Verification items for the finished model (mm, model axes). A direction names the side the tool comes from. Give positions to 0.01 mm unless a question says otherwise; leave off trailing zeros. Loops run counter-clockwise (first coordinate to the right, second up) from the corner with the lowest first, then second, coordinate; pieces in that order, holes last. Notation, with made-up numbers: M 64.5,81 L 99.5,81 A6 ccw 99.5,89 Z; hole C 15.5,6.25 d3. An arc over 180 degrees is marked long. Use a Markdown table: item, result.
from build123d import *

# Parameters (mm, degrees)
SKETCH1_W           = 30
SKETCH1_H           = 30
BOSS_EXTRUDE1_DEPTH = 150
SKETCH2_R           = 12.5
CUT_EXTRUDE1_DEPTH  = 120
SKETCH3_W           = 10
SKETCH3_H           = 5
BOSS_EXTRUDE2_DEPTH = 15
SKETCH4_R           = 2.5
CUT_EXTRUDE2_DEPTH  = 10


with BuildPart() as part:
    # Sketch1 → Boss-Extrude1 (new body)
    with BuildSketch(Plane.XY):
        with Locations((-15, 15)):
            Rectangle(SKETCH1_W, SKETCH1_H)
    extrude(amount=BOSS_EXTRUDE1_DEPTH)

    # Sketch2 → Cut-Extrude1 (cut)
    with BuildSketch(Plane.XY.offset(150)):
        with Locations((-14.468504341, 15)):
            Circle(SKETCH2_R)
    extrude(amount=-CUT_EXTRUDE1_DEPTH, mode=Mode.SUBTRACT)

    # Sketch3 → Boss-Extrude2 (add)
    with BuildSketch(Plane(origin=(0, 0, 0), x_dir=(-1, 0, 0), z_dir=(0, 0, -1))):
        with Locations((15, 15)):
            Rectangle(SKETCH3_W, SKETCH3_H)
    extrude(amount=BOSS_EXTRUDE2_DEPTH)

    # Sketch4 → Cut-Extrude2 (cut)
    with BuildSketch(Plane.XZ.offset(-12.5)):
        with Locations(Location((-15, -10, 0), (0, 0, 270))):
            Circle(SKETCH4_R)
    extrude(amount=-CUT_EXTRUDE2_DEPTH, mode=Mode.SUBTRACT)


solid = part.part
(1) Material ranges on line 1 (X direction, y = 15.4, z = -10); line 2 (X direction, y = 16.5, z = 124.5); line 3 (Y direction, x = -16.75, z = -7.5), recorded low to high.
Results below:
| item | result |
|---|---|
| line 1 | -20 to -17.5, -12.5 to -10 |
| line 2 | -30 to -26.88, -2.06 to 0 |
| line 3 | 12.5 to 17.5 |
(2) Cross-section at C-C on x = -15. Record the cut outline in (y, z), then the cut area to 3 significant figures.
Results below:
| item | result |
|---|---|
| outline | M 0,0 L 12.5,0 L 12.5,-7.5 L 17.5,-7.5 L 17.5,0 L 30,0 L 30,150 L 27.49,150 L 27.49,30 L 2.51,30 L 2.51,150 L 0,150 Z; M 12.5,-15 L 17.5,-15 L 17.5,-12.5 L 12.5,-12.5 Z |
| area | 1,550 mm^2 |
(3) Draft check along Y on faces 5 (the flat face through (-15, 17.5, -7)), 6 (the cylindrical face through (-2.922, 10.212, 90.84)), 7 (the flat face through (-15, 15, -15)). Enter one of: +Y half, -Y half, draft (parallel to the pull), parting line (faces both ways), or undercut.
Results below:
| item | result |
|---|---|
| face 5 | +Y half |
| face 6 | undercut |
| face 7 | draft |
(4) Set-up check for faces 1 (the flat face through (-15, 12.5, -7)), 2 (the flat face through (-15, 15, 30)), 3 (the flat face through (-20, 15, -7)), 4 (the flat face through (-10, 15, -7)): record each of +Z, -Z, +X, -X, +Y, -Y from which the full face is reachable in a straight line by a thin tool's end or side.
Results below:
| item | result |
|---|---|
| face 1 | -Z, +X, -X, -Y |
| face 2 | +Z |
| face 3 | -Z, -X, +Y, -Y |
| face 4 | -Z, +X, +Y, -Y |
(5) Gauge pin test, flat ends, axial feed: P1, Ø2.5, axis at y = 15.5, z = -8.5, coming from the -X side; P2, Ø5, axis at x = -13.5, z = -11, coming from the +Y side; P3, Ø3, axis at x = -4, y = 12.5, coming from the -Z side. Record the tip position at first contact, or that the pin passes through.
Results below:
| item | result |
|---|---|
| P1 | x = -20 |
| P2 | y = 17.5 |
| P3 | z = 0 |
(6) Cross-section at D-D on z = 59.5. Record the cut outline in (x, y), then the cut area to 3 significant figures.
Results below:
| item | result |
|---|---|
| outline | M -30,0 L 0,0 L 0,30 L -30,30 Z; hole C -14.47,15 d25 |
| area | 409 mm^2 |
(7) Cross-section at B-B on z = -10. Record the cut outline in (x, y).
Results below:
| item | result |
|---|---|
| outline | M -20,12.5 L -17.5,12.5 L -17.5,17.5 L -20,17.5 Z; M -12.5,12.5 L -10,12.5 L -10,17.5 L -12.5,17.5 Z |
(8) Cross-section at A-A on y = 15. Record the cut outline in (x, z), then the cut area to 3 significant figures.
Results below:
| item | result |
|---|---|
| outline | M -30,0 L -20,0 L -20,-15 L -10,-15 L -10,0 L 0,0 L 0,150 L -1.97,150 L -1.97,30 L -26.97,30 L -26.97,150 L -30,150 Z; hole C -15,-10 d5 |
| area | 1,630 mm^2 |
